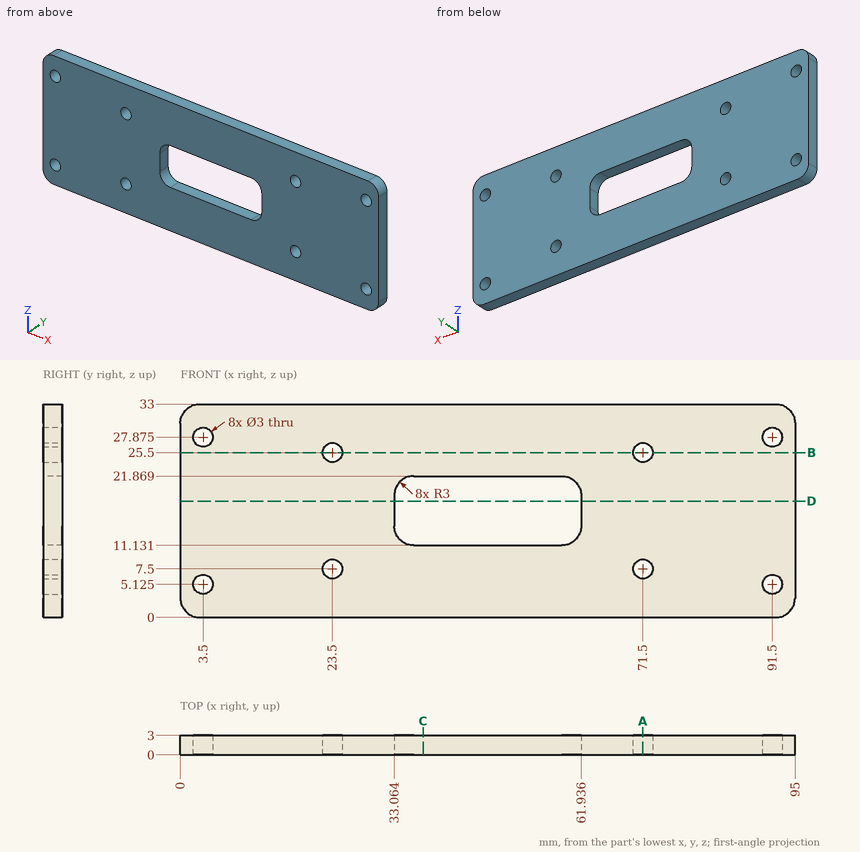
Study the drawing (mm; zero at the part's minimum x, y, z) and answer. Round coordinates to 2 decimals unless told otherwise and drop trailing zeros. Write each loop counter-clockwise with the first axis right and the second up, starting at its lowest first coordinate (ties: lowest second). Pieces come first, ordered by that corner, then holes. Notation, with made-up numbers: (47, -21.75) -> (81, -21.75) arc R26 cw to (81, -2.75) -> close; hole circle Ø11 at (81.5, -2). An arc over 180 degrees is marked (long way). Write each question's results on one line, items separated by ' | '.
Item 1: A cutting plane is placed at A-A, the plane x = 71.5. Determine the outline of the cut face in (y, z), plus the area to 3 significant figures.
Result set:
outline: (0, 0) -> (3, 0) -> (3, 6) -> (0, 6) -> close; (0, 9) -> (3, 9) -> (3, 24) -> (0, 24) -> close; (0, 27) -> (3, 27) -> (3, 33) -> (0, 33) -> close | area: 81.0 mm^2
Item 2: A cutting plane is placed at D-D, the plane z = 18. Determine the outline of the cut face in (x, y), plus the area to 3 significant figures.
Result set:
outline: (0, 0) -> (33.06, 0) -> (33.06, 3) -> (0, 3) -> close; (61.94, 0) -> (95, 0) -> (95, 3) -> (61.94, 3) -> close | area: 198 mm^2
Item 3: A cutting plane is placed at B-B, the plane z = 25.5. Determine the outline of the cut face in (x, y).
Result set:
outline: (0, 0) -> (22, 0) -> (22, 3) -> (0, 3) -> close; (25, 0) -> (70, 0) -> (70, 3) -> (25, 3) -> close; (73, 0) -> (95, 0) -> (95, 3) -> (73, 3) -> close
Item 4: Find the intervals of material crossed by line 1 along Z through (x, y) = (3.5, 1.5) (1 decimal); line 2 along X through (y, z) = (0.85, 7.5); line 3 along X through (y, z) = (2.15, 17), in increasing order. Write a range as [from, to].
Result set:
line 1: [0, 3.6], [6.6, 26.4], [29.4, 33] | line 2: [0, 22], [25, 70], [73, 95] | line 3: [0, 33.06], [61.94, 95]
Item 5: A cutting plane is placed at C-C, the plane x = 37.5. Determine the outline of the cut face in (y, z).
Result set:
outline: (0, 0) -> (3, 0) -> (3, 11.13) -> (0, 11.13) -> close; (0, 21.87) -> (3, 21.87) -> (3, 33) -> (0, 33) -> close
Item 6: A flat-ended cylindrical pin translates along its axis: P1, Ø2.5, axis at x = 23.5, z = 7.5, coming from the +Y side. Find the tip coordinate at first contact, or state that the pin passes through.
Result set:
P1: through
